from build123d import *

# Parameters (mm, degrees)
BASE_FLANGE1_DEPTH = 40
SKETCH7_R          = 4.5
CUT_EXTRUDE1_DEPTH = 2
CUT_EXTRUDE2_DEPTH = 2


# Sheet-metal steps are written as plain solids
with BuildPart() as part:
    # Sketch1 → Base-Flange1 (new body)
    with BuildSketch(Plane(origin=(0, 0, 0), x_dir=(0, 0, -1), z_dir=(1, 0, 0))):
        with BuildLine():
            Line((0, 0), (399.171572875, 0))
            ThreePointArc((399.171572875, 0), (399.93693974, 0.152240935), (400.585786438, 0.585786438))
            Line((400.585786438, 0.585786438), (449.497474683, 49.497474683))
            Line((449.497474683, 49.497474683), (450.911688245, 48.083261121))
            Line((450.911688245, 48.083261121), (402, -0.828427125))
            ThreePointArc((402, -0.828427125), (400.702306605, -1.69551813), (399.171572875, -2))
            Line((399.171572875, -2), (0, -2))
            Line((0, -2), (0, 0))
        make_face()
    extrude(amount=BASE_FLANGE1_DEPTH)

    # Sketch7 → Cut-Extrude1 (cut)
    with BuildSketch(Plane(origin=(0, -200, -200), x_dir=(1, 0, 0), z_dir=(0, 0.7071067811865456, 0.7071067811865496))):
        with Locations(Location((20, 317.842712475, 0), (0, 0, 270))):
            Circle(SKETCH7_R)
    extrude(amount=-CUT_EXTRUDE1_DEPTH, mode=Mode.SUBTRACT)

    # Sketch8 → Cut-Extrude2 (cut)
    with BuildSketch(Plane(origin=(0, 0, 0), x_dir=(1, 0, 0), z_dir=(0, 1, 0))):
        with BuildLine():
            Line((24, 50), (24, 250))
            ThreePointArc((24, 250), (20, 254), (16, 250))
            Line((16, 250), (16, 50))
            ThreePointArc((16, 50), (20, 46), (24, 50))
        make_face()
    extrude(amount=-CUT_EXTRUDE2_DEPTH, mode=Mode.SUBTRACT)


solid = part.part
Input: part model. Units: mm. Frame: model coordinates. A direction names the side the tool comes from. Give positions to 0.01 mm unless a question says otherwise; leave off trailing zeros. Order: outer loops, then holes, each group sorted by start corner. A loop starts at its lowest first (then second) coordinate and runs counter-clockwise, first axis right, second up. Notation, with made-up numbers: M 24,47 L 34,47 A10 cw 34,58 Z; hole C -19,82.5 d4. An arc over 180 degrees is marked long. Answer as a JSON object with one key per item and string values.
1. Cut plane A-A, the plane x = 7.5. Output: boundary loops of the cut face in (y, z).
Result sheet:
{"outline": "M -2,-399.17 A4 ccw -0.83,-402 L 48.08,-450.91 L 49.5,-449.5 L 0.59,-400.59 A2 cw 0,-399.17 L 0,0 L -2,0 Z"}
2. First-contact query: P1, Ø12, axis at x = 29, z = -127, coming from the +Y side; P2, Ø4, axis at x = 9.5, y = 36, coming from the +Z side; P3, Ø5, axis at x = 27.5, y = 40.5, coming from the +Z side; P4, Ø1, axis at y = -1, z = -151.5, coming from the -X side. Flat tips, straight axial feed; report the tip coordinate or a pass-through.
Result sheet:
{"P1": "y = 0", "P2": "z = -434", "P3": "z = -438", "P4": "x = 0"}
3. Cut plane B-B, the plane y = 43.5. Output: boundary loops of the cut face in (x, z).
Result sheet:
{"outline": "M 0,-446.33 L 40,-446.33 L 40,-443.5 L 0,-443.5 Z"}
4. Ray query, line 1 (Y direction, x = 9.5, z = -178.5); line 2 (Z direction, x = 36, y = 4.5); line 3 (Z direction, x = 33, y = 37). Return the intervals inside material, ascending. Write a range as [from, to].
Result sheet:
{"line 1": "[-2, 0]", "line 2": "[-407.33, -404.5]", "line 3": "[-439.83, -437]"}
5. Pull-direction query (X, two-part tool) for faces 3 (the cylindrical face through (20.198, 27.23, -428.625)), 4 (the flat face through (0, -1, -227)), 5 (the flat face through (15, -2, -202)); classes: +X half, -X half, draft (parallel to the pull), parting line (faces both ways), or undercut.
Result sheet:
{"face 3": "undercut", "face 4": "-X half", "face 5": "draft"}
6. Reachability of faces 1 (the flat face through (15, 0, -197)), 2 (the flat face through (40, -1, -227)) from +Z, -Z, +X, -X, +Y, -Y: full face, straight path, thin tool, end or side. Return the list, or none.
Result sheet:
{"face 1": "+Z, +X, -X, +Y", "face 2": "+Z, -Z, +X, +Y, -Y"}
